Autodesk Inventor part; units mm, degrees
ref_plane "Plano de trabajo2" through (-10, 32, 0) normal (0, 0, 1) x (1, 0, 0)
ref_plane "YZ Plane" through (0, 0, 0) normal (1, 0, 0) x (0, 1, 0)
ref_plane "XZ Plane" through (0, 0, 0) normal (0, 1, 0) x (-1, 0, 0)
sketch "Boceto1" plane through (0, 0, 0) normal (0, 1, 0) x (-1, 0, 0)
  circle A0 centre (0, 0) radius 15
  dimension "d0" = 30
extrude "Extrusión1" add sketch "Boceto1" along normal blind 30
sketch "Boceto4" plane through (0, 30, 0) normal (0, 1, 0) x (1, 0, 0)
  circle A0 centre (0, 0) radius 10
  dimension "d7" = 20
extrude "Extrusión2" add sketch "Boceto4" along normal blind 2
sketch "Boceto5" plane through (0, 32, 0) normal (0, 1, 0) x (1, 0, 0)
  circle A0 centre (0, 0) radius 10
  line L0 (-10, 0) -> (10, 0)
ref_plane "Plano de trabajo2" through (-10, 32, 0) normal (0, 0, 1) x (1, 0, 0)
sketch "Boceto6" plane through (-10, 32, 0) normal (0, 0, 1) x (1, 0, 0)
  line L0 (20, 0) -> (0, 0)
  circle A0 centre (10, 0) radius 6
  line L1 (4, 0) -> (16, 0)
  point P0 (10, -32)
  dimension "d11" = 12
revolve "Revolución2" add sketch "Boceto6" angle 360 about axis through (-6, 32, 0) along (1, 0, 0) picked at (11.497, 2.2835) contours L0 A0
sketch "Boceto7" plane through (0, 0, 0) normal (0, -1, 0) x (1, 0, 0)
  circle A0 centre (0, 0) radius 7.5
  dimension "d13" = 15
extrude "Extrusión3" add sketch "Boceto7" along normal blind 65
properties part number "Rodillo_Sostener"
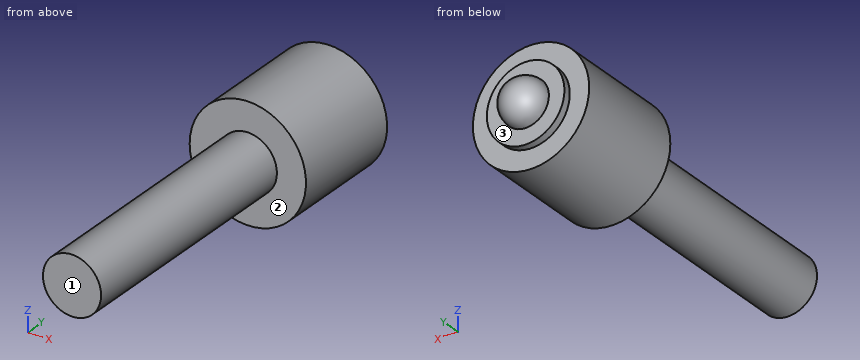
Geometry check sheet. Reference: the model listing, model coordinates, mm. Face numbers are marked on the shaded views. A direction names the side the tool comes from. Give positions to 0.01 mm unless a question says otherwise; leave off trailing zeros. Write each loop counter-clockwise with the first axis right and the second up, starting at its lowest first coordinate (ties: lowest second). Pieces come first, ordered by that corner, then holes. Notation, with made-up numbers: (25.5, 81) -> (50.5, 81) arc R28 ccw to (50.5, 119) -> close; hole circle Ø5 at (28.5, -22). An arc over 180 degrees is marked (long way). One line per question, with ' | ' between items.
Item 1: Scan lines: line 1 along Y through (x, z) = (5.25, -6.5); line 2 along Y through (x, z) = (-10.5, -9.5); line 3 along Z through (x, y) = (-3.25, -45). Record each from-to range of solid material in increasing order.
Determined:
line 1: 0 to 32 | line 2: 0 to 30 | line 3: -6.76 to 6.76
Item 2: Sectioned sample at B-B, the plane x = 0. Record the boundary of the cut face in (y, z), plus the area to 3 significant figures.
Determined:
outline: (-65, -7.5) -> (0, -7.5) -> (0, -15) -> (30, -15) -> (30, -10) -> (32, -10) -> (32, -6) arc R6 ccw to (32, 6) -> (32, 10) -> (30, 10) -> (30, 15) -> (0, 15) -> (0, 7.5) -> (-65, 7.5) -> close | area: 1,970 mm^2
Item 3: Sectioned sample at A-A, the plane z = 0. Record the boundary of the cut face in (x, y).
Determined:
outline: (-15, 0) -> (-7.5, 0) -> (-7.5, -65) -> (7.5, -65) -> (7.5, 0) -> (15, 0) -> (15, 30) -> (10, 30) -> (10, 32) -> (6, 32) arc R6 ccw to (-6, 32) -> (-10, 32) -> (-10, 30) -> (-15, 30) -> close
Item 4: Sectioned sample at C-C, the plane y = 11.5. Record the boundary of the cut face in (x, z).
Determined:
outline: circle Ø30 at (0, 0)
Item 5: Depth check by flat-ended pin: pin 1 (12 mm diameter, centred on x = 11, z = -6.5, fed in from +Y); pin 2 (8 mm diameter, centred on x = 0.5, z = 7, fed in from +Y); pin 3 (4 mm diameter, centred on x = -3, z = 0.5, fed in from +Y). Enter the tip coordinate at first touch or a pass-through.
Determined:
pin 1: y = 32 | pin 2: y = 37.19 | pin 3: y = 37.91
Item 6: Access from +Z, -Z, +X, -X, +Y, -Y to the whole of each face (thin tool, end or side, straight path). Record for the marked faces 1, 2 and 3.
Determined:
face 1: +Z, -Z, +X, -X, -Y | face 2: -Y | face 3: +Y
Item 7: Sectioned sample at D-D, the plane y = -50.5. Record the boundary of the cut face in (x, z).
Determined:
outline: circle Ø15 at (0, 0)
